Verification items for the finished model (mm, model axes). A direction names the side the tool comes from. Coordinates: 2 decimals unless noted, no trailing zeros. Write item = value, one per line. Start each with the question number.
from build123d import *

# Parameters (mm, degrees)
SKETCH1_R           = 75
BOSS_EXTRUDE1_DEPTH = 3
SKETCH2_R           = 1.75
CUT_EXTRUDE1_DEPTH  = 107.108435103
SKETCH3_R           = 40.5
SKETCH3_R_2         = 37.5
BOSS_EXTRUDE2_DEPTH = 3
SKETCH4_W           = 3
SKETCH4_H           = 30
CUT_EXTRUDE2_DEPTH  = 107.235587258


with BuildPart() as part:
    # Sketch1 → Boss-Extrude1 (new body)
    with BuildSketch(Plane.XY):
        Circle(SKETCH1_R)
    extrude(amount=BOSS_EXTRUDE1_DEPTH)

    # Sketch2 → Cut-Extrude1 (cut, through all)
    with BuildSketch(Plane.XY.offset(3)):
        with Locations((-50, 15)):
            Circle(SKETCH2_R)
        with Locations((-50, -15)):
            Circle(SKETCH2_R)
        with Locations((50, -15)):
            Circle(SKETCH2_R)
        with Locations((50, 15)):
            Circle(SKETCH2_R)
        Circle(SKETCH2_R)
    extrude(amount=-CUT_EXTRUDE1_DEPTH, mode=Mode.SUBTRACT)

    # Sketch3 → Boss-Extrude2 (add)
    with BuildSketch(Plane.XY.offset(3)):
        Circle(SKETCH3_R)
        Circle(SKETCH3_R_2, mode=Mode.SUBTRACT)
    extrude(amount=BOSS_EXTRUDE2_DEPTH)

    # Sketch4 → Cut-Extrude2 (cut, through all)
    with BuildSketch(Plane(origin=(0, 0, 0), x_dir=(-1, 0, 0), z_dir=(0, 0, -1))):
        with Locations((-26.5, -50)):
            Rectangle(SKETCH4_W, SKETCH4_H)
        with Locations((26.5, -50)):
            Rectangle(SKETCH4_W, SKETCH4_H)
    extrude(amount=-CUT_EXTRUDE2_DEPTH, mode=Mode.SUBTRACT)

    # Sketch5 → Revolve1 (revolve)
    with BuildSketch(Plane(origin=(0, 0, 0), x_dir=(1, 0, 0), z_dir=(0, 1, 0)), mode=Mode.PRIVATE) as revolve1_sk:
        Polygon((-75, 0), (-80.773502692, -10), (-78.464101615, -10), (-72.690598923, 0), align=None)
    revolve(revolve1_sk.sketch.rotate(Axis((0, 0, 0), (0, 0, 1)), 180), axis=Axis((0, 0, 0), (0, 0, 1)))


solid = part.part
Item 1: Thickness scan on line 1 (Y direction, x = 50, z = 1.4); line 2 (Y direction, x = 50, z = 1.8); line 3 (Z direction, x = -55, y = 25). Record the ranges inside material, lowest first.
Item 2: Tool access check on faces 1 (the cylindrical face through (-48.331, 15.526, 1.521)), 2 (the cylindrical face through (-4.88, 37.18, 4.48)). Record the directions out of +Z, -Z, +X, -X, +Y, -Y that give a thin tool (end or side, any length) a straight path to the whole face; none if there is none.
Item 3: Section check A-A (y = -58). State how many separate pieces and enclosed holes the cut face has, then the cut area to 3 significant figures.
Item 4: Gauge pin test, flat ends, axial feed: P1, Ø3.5, axis at x = -27, z = 2, coming from the -Y side; P2, Ø3.5, axis at y = -48, z = 1, coming from the +X side; P3, Ø8, axis at x = -63.5, y = -53.5, coming from the -Z side. Record the tip position at first contact, or that the pin passes through.
Item 5: Mould release check, pull along X, two halves, no side actions. Record for faces 3 (the flat face through (16, 1, 0)), 4 (the conical face through (34.775, -66.858, 0.626)), 5 (the cylindrical face through (1.617, -0.67, 1.521)): pulls with the +X half, pulls with the -X half, needs draft (parallel to the pull), parting line crosses it, or undercut.
Filled sheet:
q1.line_1 = -56.98 to -16.75, -13.25 to 13.25, 16.75 to 56.98
q1.line_2 = -57.29 to -16.75, -13.25 to 13.25, 16.75 to 57.29
q1.line_3 = 0 to 3
q2.face_1 = +Z, -Z
q2.face_2 = +Z
q3.separate_pieces = 3
q3.enclosed_holes = 0
q3.area = 324 mm^2
q4.P1 = -72.46
q4.P2 = 60.28
q4.P3 = 6.99
q5.face_3 = needs draft
q5.face_4 = parting line crosses it
q5.face_5 = undercut
